Autodesk Inventor part; units mm, degrees
ref_plane "YZ Plane" through (0, 0, 0) normal (1, 0, 0) x (0, 1, 0)
ref_plane "XZ Plane" through (0, 0, 0) normal (0, 1, 0) x (-1, 0, 0)
ref_plane "XY Plane" through (0, 0, 0) normal (0, 0, 1) x (1, 0, 0)
sketch "Sketch1" plane through (0, 0, 0) normal (0, 1, 0) x (-1, 0, 0)
  line L0 (-10.16, 10.16) -> (10.16, 10.16)
  line L1 (10.16, 10.16) -> (10.16, -10.16)
  line L2 (-10.16, -10.16) -> (-10.16, 10.16)
  circle A0 centre (6.9088, -6.9148) radius 1.9304
  circle A1 centre (6.9148, 6.9148) radius 1.9304
  circle A2 centre (-6.9148, 6.9148) radius 1.9304
  circle A3 centre (-6.9088, -6.9148) radius 1.9304
  line L3 (-5.715, -10.16) -> (-5.715, -19.939)
  line L4 (-5.715, -19.939) -> (6.985, -19.939)
  line L5 (6.985, -19.939) -> (6.985, -10.16)
  line L6 (10.16, -10.16) -> (6.985, -10.16)
  line L7 (-5.715, -10.16) -> (-10.16, -10.16)
  point P0 (0, 0)
  dimension "d0" = 20.32
  dimension "d2" = 10.16
  dimension "d3" = 10.16
  dimension "d4" = 3.8608
  dimension "d5" = 6.9148
  dimension "d6" = 6.9088
  dimension "d7" = 3.8608
  dimension "d8" = 6.9148
  dimension "d9" = 6.9148
  dimension "d10" = 3.8608
  dimension "d11" = 6.9148
  dimension "d12" = 6.9148
  dimension "d13" = 3.8608
  dimension "d14" = 12.7
  dimension "d16" = 6.985
  dimension "d43" = 10.16
  dimension "d44" = 10.16
  dimension "d45" = 6.9148
  dimension "d46" = 9.779
  dimension "d47" = 9.779
extrude "Extrusion1" add sketch "Sketch1" along normal blind 6.985
sketch "Sketch2" plane through (-6.985, 0, -19.939) normal (-1, 0, 0) x (0, 0, 1)
  circle A0 centre (5.08, 3.4925) radius 4.6609 construction
  line L0 (9.779, 0) -> (0, 0)
  line L1 (0, 0) -> (0, 6.985)
  line L2 (9.7409, 3.4925) -> (7.4105, -0.544)
  line L3 (7.4105, -0.544) -> (2.7496, -0.544)
  line L4 (2.7496, -0.544) -> (0.4191, 3.4925)
  line L5 (0.4191, 3.4925) -> (2.7495, 7.529)
  line L6 (2.7495, 7.529) -> (7.4104, 7.529)
  line L7 (7.4104, 7.529) -> (9.7409, 3.4925)
  point P0 (19.939, 0)
  dimension "d19" = 9.3218
  dimension "d20" = 3.4925
  dimension "d21" = 5.08
extrude "Extrusion2" cut sketch "Sketch2" against normal blind 3.81
sketch "Sketch3" plane through (5.715, 0, -10.16) normal (1, 0, 0) x (0, 0, -1)
  circle A0 centre (4.699, 3.4925) radius 1.9304
  line L0 (9.779, 0) -> (9.779, 6.985)
  line L1 (0, 6.985) -> (9.779, 6.985)
  point P0 (-10.16, 0)
  dimension "d24" = 3.8608
  dimension "d25" = 5.08
  dimension "d26" = 3.4925
extrude "Extrusion3" cut sketch "Sketch3" against normal through all
sketch "Sketch4" plane through (0, 6.985, 0) normal (0, 1, 0) x (1, 0, 0)
  circle A0 centre (0, 0) radius 6.35
  dimension "d29" = 12.7
extrude "Extrusion4" add sketch "Sketch4" along normal blind 2.54
sketch "Sketch5" plane through (0, 9.525, 0) normal (0, 1, 0) x (1, 0, 0)
  arc A0 (2.0472, -2.5908) -> (-2.0472, -2.5908) centre (0, 0) ccw
  line L0 (-2.0472, -2.5908) -> (2.0472, -2.5908)
  dimension "d32" = 6.604
  dimension "d33" = 2.5908
fillet "Fillet1" radius 3.3782 4 edges at (10.16, 3.4925, 10.16) (10.16, 3.4925, -10.16) (-10.16, 3.4925, 10.16) (-10.16, 3.4925, -10.16)
extrude "Extrusion5" cut sketch "Sketch5" against normal through all
sketch "Sketch6" plane through (0, 9.525, 0) normal (0, 1, 0) x (1, 0, 0)
  line L0 (-6.985, 19.939) -> (5.715, 19.939)
  line L1 (0.4649, 0) -> (0.4649, 19.939)
  line L2 (0.4649, 19.939) -> (-0.635, 20.574)
  line L3 (-0.635, 20.574) -> (-0.635, 0)
  line L4 (-0.4947, -21.2174) -> (0.4649, 19.939) construction
  line L5 (0.635, -20.574) -> (-0.635, 20.574) construction
  line L6 (-0.635, 0) -> (0.4649, 0)
  point P0 (0, 0)
  dimension "d37" = 1.27
extrude "Extrusion6" cut sketch "Sketch6" against normal through all
sketch "Sketch7" plane through (0, 0, 0) normal (0, -1, 0) x (1, 0, 0)
  circle A0 centre (-6.9148, 6.9148) radius 1.9304 construction
  circle A1 centre (-6.9148, 6.9148) radius 4.6609 construction
  point P0 (0, 0)
  dimension "d40" = 9.3218
properties part number "clamping hub 1_4 D through holes"
For this review, take the finished solid that the model builds, in its own axes (mm). A direction names the side the tool comes from. Round coordinates to 2 decimals unless told otherwise and drop trailing zeros. Write each loop counter-clockwise with the first axis right and the second up, starting at its lowest first coordinate (ties: lowest second). Pieces come first, ordered by that corner, then holes. Notation, with made-up numbers: (5, 33) - (24, 33) arc R30 cw to (24, 57) - close; hole circle Ø3 at (-32.75, 47). An arc over 180 degrees is marked (long way). Answer as a JSON object with one key per item and string values.
1. Draft analysis for pull direction X (two halves, no side actions). For faces 6 (the face through (5.877, 3.444, 5.287)), 7 (the face through (9.2, 3.44, 9.14)), 8 (the face through (-4, 3, -19.939)), 9 (the face through (3.2, 4.83, -0.81)), state which applies: +X half, -X half, draft (parallel to the pull), parting line (faces both ways), or undercut.
Response values:
{"face 6": "undercut", "face 7": "+X half", "face 8": "draft", "face 9": "undercut"}
2. We need section A-A on y = 4. Count the separate pieces of the cut face and the enclosed holes in it, then the cut area to 3 significant figures.
Response values:
{"separate pieces": "3", "enclosed holes": "4", "area": "368 mm2"}
3. To check wall thickness, follow line 1 along X through (y, z) = (6, 7); line 2 along X through (y, z) = (6, -13) (3 decimals); line 3 along Z through (x, y) = (0.5, 6.75). State the ranges of each line that lie inside material, in increasing order.
Response values:
{"line 1": "x = -10.15 to -8.84, -4.99 to 4.99, 8.84 to 10.15", "line 2": "x = -3.175 to -0.635, 0.465 to 5.715", "line 3": "z = -19.94 to -3.26, 2.59 to 10.16"}
4. We need section D-D on x = 7.75. Give the boundary of the cut face in (y, z) (3 decimals), then the cut area to 3 significant figures.
Response values:
{"outline": "(0, -10.018) - (6.985, -10.018) - (6.985, -8.652) - (0, -8.652) - close; (0, -5.177) - (6.985, -5.177) - (6.985, 5.174) - (0, 5.174) - close; (0, 8.655) - (6.985, 8.655) - (6.985, 10.018) - (0, 10.018) - close", "area": "91.4 mm2"}
5. Tool access review of faces 1 (the face through (5.715, 3, -17)), 2 (the face through (-6.985, 5, -10.7)), 3 (the face through (-3.175, 4, -17)), 4 (the face through (0.36, 8.24, 6.34)), 5 (the face through (-0.635, 4, -12)): name each direction out of +Z, -Z, +X, -X, +Y, -Y from which nothing blocks a thin tool from reaching the whole face with its end or side.
Response values:
{"face 1": "-Z, +X, +Y, -Y", "face 2": "-Z, -X, +Y, -Y", "face 3": "-X", "face 4": "+Y", "face 5": "-Z, +Y, -Y"}
6. We need section C-C on x = -5.75. Give the boundary of the cut face in (y, z) (1 decimal).
Response values:
{"outline": "(0, -19.9) - (7, -19.9) - (7, -17.5) - (3.5, -19.5) - (0, -17.5) - close; (0, -12.2) - (3.5, -10.2) - (7, -12.2) - (7, -8.5) - (0, -8.5) - close; (0, -5.4) - (7, -5.4) - (7, -2.7) - (9.5, -2.7) - (9.5, 2.7) - (7, 2.7) - (7, 5.4) - (0, 5.4) - close; (0, 8.5) - (7, 8.5) - (7, 10.2) - (0, 10.2) - close"}
7. We need section B-B on z = 0. Give the boundary of the cut face in (x, y) (3 decimals).
Response values:
{"outline": "(-10.16, 0) - (-3.302, 0) - (-3.302, 9.525) - (-6.35, 9.525) - (-6.35, 6.985) - (-10.16, 6.985) - close; (3.302, 0) - (10.16, 0) - (10.16, 6.985) - (6.35, 6.985) - (6.35, 9.525) - (3.302, 9.525) - close"}
8. For pin 1 Ø2 at (y, z) = (5.5, -14) entering from +X (3 decimals); pin 2 Ø6 at (x, z) = (-6.91, -6.91) entering from +Y (3 decimals); pin 3 Ø0.5 at (x, y) = (6, 4) entering from -Z; pin 4 Ø3 at (x, z) = (6.91, -6.91) entering from +Y, all flat-tipped, find the tip position at first contact; note any pin that passes through.
Response values:
{"pin 1": "stops at x = 5.715", "pin 2": "stops at y = 6.985", "pin 3": "stops at z = -10.16", "pin 4": "passes through"}
